from build123d import *

# Parameters (mm, degrees)
F0_R     = 15.7
F0_R_2   = 12.7
F1_DEPTH = 50
F4_R     = 12.7
F5_DEPTH = 6
F7_DEPTH = 1.5
F9_DEPTH = 1.5
F10_R    = 5
F11_R    = 3


with BuildPart() as f1:
    # F0 (on Top) → F1 (new body)
    with BuildSketch(Plane.XY):
        Circle(F0_R)
        Circle(F0_R_2, mode=Mode.SUBTRACT)
    extrude(amount=F1_DEPTH)

    # F2 (on Right) → F3 (revolve)
    with BuildSketch(Plane.YZ):
        Polygon((22.7, 12.5), (15.7, 12.5), (15.7, 0), (77.5868, -75), (84.5868, -75), align=None)
    revolve(axis=Axis((0, 0, -38.817684), (0, 0, -1)))

    # F4 (on face) → F5 (join)
    with BuildSketch(Plane(origin=(0, 0, 0), x_dir=(1, 0, 0), z_dir=(0, 0, -1))):
        Circle(F4_R)
    extrude(amount=-F5_DEPTH)

    # F6 (on Right) → F7 (join, symmetric)
    with BuildSketch(Plane.YZ):
        Polygon((77.5868, -75), (15.7, 0), (0, 0), (-15.7, 0), (-77.5868, -75), (0, -75), align=None)
    extrude(amount=F7_DEPTH, both=True)

    # F8 (on Front) → F9 (join, symmetric)
    with BuildSketch(Plane.XZ):
        Polygon((77.5868, -75), (15.7, 0), (-15.7, 0), (-77.5868, -75), (0, -75), align=None)
    extrude(amount=F9_DEPTH, both=True)

    # F10
    f10_edges = [f1.edges().sort_by_distance(p)[0] for p in [
        (0, -22.7, 12.5),
    ]]
    fillet(f10_edges, radius=F10_R)

    # F11
    f11_edges = [f1.edges().sort_by_distance(p)[0] for p in [
        (0, -84.5868, -75),
    ]]
    fillet(f11_edges, radius=F11_R)


solid = f1.part
Design review of the part built by this model. Coordinates are the model's own, in mm. A direction names the side the tool comes from. Coordinates: 2 decimals unless noted, no trailing zeros. Loops run counter-clockwise (first coordinate to the right, second up) from the corner with the lowest first, then second, coordinate; pieces in that order, holes last. Notation, with made-up numbers: M 54,51.25 L 109,51.25 A27 cw 109,85.25 Z; hole C 28,-22 d3. An arc over 180 degrees is marked long. Use one line per item in the form item = value.
(1) For line 1 along Y through (x, z) = (0, 22.5); line 2 along Y through (x, z) = (-3, -27.5), list the stretches that pass through material, from the lowest coordinate up. Write a range as from..to.
Return value:
line_1 = -15.7..-12.7, 12.7..15.7
line_2 = -50.9..-38.27, -1.5..1.5, 38.27..50.9
(2) For faces 1 (the face through (13, 0, 50)), 2 (the face through (-2.75, -12.4, 27.69)), 3 (the face through (32.93, 33.64, -38.02)), list the 3-axis set-ups (+Z, -Z, +X, -X, +Y, -Y) from which the entire face can be reached by the end or side of a thin tool; tool diameter is ignored.
Return value:
face_1 = +Z, +X, -X, +Y, -Y
face_2 = +Z
face_3 = -Z
(3) Consider section B-B (z = -41). Write out the cut boundary in (x, y).
Return value:
outline = C 0,0 d121.08; hole M -49.51,-1.5 A49.53 ccw -1.5,-49.51 L -1.5,-1.5 Z; hole M -49.51,1.5 L -1.5,1.5 L -1.5,49.51 A49.53 ccw Z; hole M 1.5,-49.51 A49.53 ccw 49.51,-1.5 L 1.5,-1.5 Z; hole M 1.5,1.5 L 49.51,1.5 A49.53 ccw 1.5,49.51 Z
(4) Draft analysis for pull direction X (two halves, no side actions). For faces 4 (the face through (1.5, -32, -45)), 5 (the face through (-12.76, 30.76, -2.49)), 6 (the face through (0, 0, -75)), state which applies: pulls with the +X half, pulls with the -X half, needs draft (parallel to the pull), parting line crosses it, or undercut.
Return value:
face_4 = undercut
face_5 = parting line crosses it
face_6 = needs draft
(5) Clearance check with flat-ended pins moving along their axes: P1, Ø20.5, axis at x = 0, y = 0, coming from the +Z side; P2, Ø1.5, axis at x = 0, z = -3.5, coming from the -Y side; P3, Ø11.5, axis at x = -8.5, y = 5.5, coming from the -Z side; P4, Ø1.5, axis at x = -47, y = -56, coming from the -Z side. State where each tip first meets the part, or that it passes through.
Return value:
P1 = 6
P2 = -34.55
P3 = -75
P4 = -70.48
(6) Consider section A-A (z = 31.5). Write out the cut boundary in (x, y), and give its area (3 significant figures).
Return value:
outline = C 0,0 d31.4; hole C 0,0 d25.4
area = 268 mm2
